Design review of the part built by this model. Coordinates are the model's own, in mm. A direction names the side the tool comes from. Round coordinates to 2 decimals unless told otherwise and drop trailing zeros. Order: outer loops, then holes, each group sorted by start corner. A loop starts at its lowest first (then second) coordinate and runs counter-clockwise, first axis right, second up. Notation, with made-up numbers: M 56,49.25 L 106,49.25 A35 cw 106,83.25 Z; hole C -20,64 d8. An arc over 180 degrees is marked long. Write each question's results on one line, items separated by ' | '. Start each with the question number.
Item 1: Machinability: for faces 1 (the flat face through (-57.785, -204.087, 4.93)), 2 (the flat face through (202.41, 344.14, 4.93)), which of the approach directions +Z, -Z, +X, -X, +Y, -Y give a long, thin tool a straight path to every point of the face, cutting with its end or side? Answer none if there is none.
Item 2: Clearance check with flat-ended pins moving along their axes: pin 1 (1 mm diameter, centred on y = 254, z = 8, fed in from -X); pin 2 (18 mm diameter, centred on x = 0, y = 0, fed in from +Z); pin 3 (3 mm diameter, centred on x = 101.5, z = 5.5, fed in from +Y) (3 decimals); pin 4 (3 mm diameter, centred on x = 274.5, z = 1.5, fed in from -Y). State where each tip first meets the part, or that it passes through.
Item 3: Take a section at C-C, the plane y = -380. Write out the cut boundary in (x, z), plus the area to 3 significant figures.
Item 4: Wall thickness on line 1 (X direction, y = -8, z = 2); line 2 (X direction, y = 11, z = 3); line 3 (Y direction, x = -84.5, z = 3.25): over which ranges is each line inside the solid? List them lowest first. Write a range as [from, to].
Item 5: The part is to be moulded in two halves that separate along Y. For faces 3 (the flat face through (-202.41, -344.14, 4.93)), 4 (the flat face through (-104.24, 240.04, 4.93)), 5 (the flat face through (-196.824, 347.364, 4.93)), say which applies: +Y half, -Y half, draft (parallel to the pull), parting line (faces both ways), or undercut.
Item 6: Take a section at A-A, the plane z = 8.5. Count the separate pieces of the cut face and the enclosed holes in it, plus the area to 3 significant figures.
Item 7: Take a section at B-B, the plane x = -343.5. Write out the cut boundary in (y, z), plus the area to 3 significant figures.
```python
from build123d import *

# Parameters (mm, degrees)
ESQUISSE1_R        = 10
ESQUISSE1_R_2      = 3
ESQUISSE1_R_3      = 2
ESQUISSE1_R_4      = 6
BOSS_EXTRU_1_DEPTH = 10


with BuildPart() as part:
    # Esquisse1 → Boss.-Extru.1 (new body)
    with BuildSketch(Plane.XY):
        Polygon((399.237711145, 230.5), (0, 461), (-399.237711145, 230.5), (-399.237711145, -230.5), (0, -461), (399.237711145, -230.5), align=None)
        Circle(ESQUISSE1_R, mode=Mode.SUBTRACT)
        with Locations((140, -29)):
            Circle(ESQUISSE1_R_2, mode=Mode.SUBTRACT)
        with Locations((140, -56.5)):
            Circle(ESQUISSE1_R_3, mode=Mode.SUBTRACT)
        with Locations((140, -84)):
            Circle(ESQUISSE1_R_2, mode=Mode.SUBTRACT)
        with Locations((378.237711145, 0)):
            Circle(ESQUISSE1_R_4, mode=Mode.SUBTRACT)
        with Locations((378.237711145, 35)):
            Circle(ESQUISSE1_R_3, mode=Mode.SUBTRACT)
        with Locations((378.237711145, -35)):
            Circle(ESQUISSE1_R_3, mode=Mode.SUBTRACT)
        with Locations((270, -84)):
            Circle(ESQUISSE1_R_2, mode=Mode.SUBTRACT)
        with Locations((270, -56.5)):
            Circle(ESQUISSE1_R_3, mode=Mode.SUBTRACT)
        with Locations((270, -29)):
            Circle(ESQUISSE1_R_2, mode=Mode.SUBTRACT)
        with Locations((-95.11473671, -106.74355653)):
            Circle(ESQUISSE1_R_2, mode=Mode.SUBTRACT)
        with Locations((-118.930435314, -92.99355653)):
            Circle(ESQUISSE1_R_3, mode=Mode.SUBTRACT)
        with Locations((-142.746133918, -79.24355653)):
            Circle(ESQUISSE1_R_2, mode=Mode.SUBTRACT)
        with Locations((-207.746133918, -191.826859022)):
            Circle(ESQUISSE1_R_2, mode=Mode.SUBTRACT)
        with Locations((-183.930435314, -205.576859022)):
            Circle(ESQUISSE1_R_3, mode=Mode.SUBTRACT)
        with Locations((-160.11473671, -219.326859022)):
            Circle(ESQUISSE1_R_2, mode=Mode.SUBTRACT)
        with Locations((-189.118855572, -327.563466521)):
            Circle(ESQUISSE1_R_4, mode=Mode.SUBTRACT)
        with Locations((-158.80796644, -345.063466521)):
            Circle(ESQUISSE1_R_3, mode=Mode.SUBTRACT)
        with Locations((-219.429744705, -310.063466521)):
            Circle(ESQUISSE1_R_3, mode=Mode.SUBTRACT)
        with Locations((-44.88526329, 135.74355653)):
            Circle(ESQUISSE1_R_2, mode=Mode.SUBTRACT)
        with Locations((-21.069564686, 149.49355653)):
            Circle(ESQUISSE1_R_3, mode=Mode.SUBTRACT)
        with Locations((2.746133918, 163.24355653)):
            Circle(ESQUISSE1_R_2, mode=Mode.SUBTRACT)
        with Locations((-62.253866082, 275.826859022)):
            Circle(ESQUISSE1_R_2, mode=Mode.SUBTRACT)
        with Locations((-86.069564686, 262.076859022)):
            Circle(ESQUISSE1_R_3, mode=Mode.SUBTRACT)
        with Locations((-109.88526329, 248.326859022)):
            Circle(ESQUISSE1_R_2, mode=Mode.SUBTRACT)
        with Locations((-189.118855572, 327.56346652)):
            Circle(ESQUISSE1_R_4, mode=Mode.SUBTRACT)
        with Locations((-219.429744705, 310.06346652)):
            Circle(ESQUISSE1_R_3, mode=Mode.SUBTRACT)
        with Locations((-158.80796644, 345.06346652)):
            Circle(ESQUISSE1_R_3, mode=Mode.SUBTRACT)
        with BuildLine():
            Line((150, 42.5), (150, -130.5))
            ThreePointArc((150, -130.5), (152.782485579, -137.217514421), (159.5, -140))
            Line((159.5, -140), (280.5, -140))
            ThreePointArc((280.5, -140), (287.217514421, -137.217514421), (290, -130.5))
            Line((290, -130.5), (290, -109.5))
            ThreePointArc((290, -109.5), (287.217514421, -102.782485579), (280.5, -100))
            Line((280.5, -100), (260, -100))
            Line((260, -100), (260, 42.5))
            ThreePointArc((260, 42.5), (257.217514421, 49.217514421), (250.5, 52))
            Line((250.5, 52), (159.5, 52))
            ThreePointArc((159.5, 52), (152.782485579, 49.217514421), (150, 42.5))
        make_face(mode=Mode.SUBTRACT)
        with BuildLine():
            Line((-80.216679003, -242.939363648), (-34.716679003, -164.131051904))
            ThreePointArc((-34.716679003, -164.131051904), (-33.767624989, -156.922270975), (-38.193920339, -151.153810568))
            Line((-38.193920339, -151.153810568), (-188.016315194, -64.653810568))
            ThreePointArc((-188.016315194, -64.653810568), (-195.225096122, -63.704756554), (-200.99355653, -68.131051904))
            Line((-200.99355653, -68.131051904), (-261.49355653, -172.920125762))
            ThreePointArc((-261.49355653, -172.920125762), (-262.442610544, -180.12890669), (-258.016315194, -185.897367098))
            Line((-258.016315194, -185.897367098), (-239.829781714, -196.397367098))
            ThreePointArc((-239.829781714, -196.397367098), (-232.621000786, -197.346421111), (-226.852540378, -192.920125762))
            Line((-226.852540378, -192.920125762), (-216.602540378, -175.166604984))
            Line((-216.602540378, -175.166604984), (-93.193920339, -246.416604984))
            ThreePointArc((-93.193920339, -246.416604984), (-85.985139411, -247.365658998), (-80.216679003, -242.939363648))
        make_face(mode=Mode.SUBTRACT)
        with BuildLine():
            Line((-170.283320997, 190.939363648), (-124.783320997, 112.131051904))
            ThreePointArc((-124.783320997, 112.131051904), (-119.014860589, 107.704756554), (-111.806079661, 108.653810568))
            Line((-111.806079661, 108.653810568), (38.016315194, 195.153810568))
            ThreePointArc((38.016315194, 195.153810568), (42.442610544, 200.922270975), (41.49355653, 208.131051904))
            Line((41.49355653, 208.131051904), (-19.00644347, 312.920125761))
            ThreePointArc((-19.00644347, 312.920125761), (-24.774903878, 317.346421111), (-31.983684806, 316.397367097))
            Line((-31.983684806, 316.397367097), (-50.170218286, 305.897367097))
            ThreePointArc((-50.170218286, 305.897367097), (-54.596513635, 300.12890669), (-53.647459622, 292.920125761))
            Line((-53.647459622, 292.920125761), (-43.397459622, 275.166604984))
            Line((-43.397459622, 275.166604984), (-166.806079661, 203.916604984))
            ThreePointArc((-166.806079661, 203.916604984), (-171.232375011, 198.148144576), (-170.283320997, 190.939363648))
        make_face(mode=Mode.SUBTRACT)
    extrude(amount=BOSS_EXTRU_1_DEPTH)


solid = part.part
```
Results list:
1) face 1: +Z, -Z | face 2: +Z, -Z, +X, +Y
2) pin 1: x = -359.4 | pin 2: through | pin 3: y = 403.265 | pin 4: y = -303.38
3) outline: M -140.3,0 L 140.3,0 L 140.3,10 L -140.3,10 Z | area: 2,810 mm²
4) line 1: [-399.24, -6], [6, 150], [260, 399.24] | line 2: [-399.24, 150], [260, 399.24] | line 3: [-412.21, -246.83], [-124.42, 124.42], [251.44, 260.84], [263.32, 412.21]
5) face 3: -Y half | face 4: undercut | face 5: +Y half
6) separate pieces: 1 | enclosed holes: 31 | area: 484,000 mm²
7) outline: M -262.68,0 L 262.68,0 L 262.68,10 L -262.68,10 Z | area: 5,250 mm²
